CAD build for the part. Positions are in the model's coordinates, mm. Face numbers are marked on the shaded views. A direction names the side the tool comes from. Round coordinates to 2 decimals unless told otherwise and drop trailing zeros. Write each loop counter-clockwise with the first axis right and the second up, starting at its lowest first coordinate (ties: lowest second). Pieces come first, ordered by that corner, then holes. Notation, with made-up numbers: (-30, 66) -> (-24, 66) arc R31 ccw to (-24, 92) -> close; hole circle Ø1 at (26.5, 14.5). An arc over 180 degrees is marked (long way). Put each result on its own line as item: value. Start each with the question number.
1. Saw through at B-B on z = 0. List the corners of the cut face in (x, y), and give its area (3 significant figures).
2. Pull direction Z, two halves, no side cores. Call the marked faces 1, 2 and 3: pulls with the +Z half, pulls with the -Z half, needs draft (parallel to the pull), parting line crosses it, or undercut.
3. Drill centre lines: line 1 (X direction, y = 1.2, z = 0); line 2 (X direction, y = 0.6, z = 1.25); line 3 (Z direction, x = 12, y = 1.6). Where is each one in solid material? Low to high. Write a range as from..to.
4. Flat gauge pins, fed straight in: P1, Ø0.9, axis at y = 2, z = 5.5, coming from the +X side; P2, Ø6, axis at x = 9, z = 1, coming from the +Y side; P3, Ø1, axis at x = 22.5, y = 1, coming from the +Z side. Where does each tip first touch, or does it go through?
5. Saw through at C-C on y = 0.55. List the corners of the cut face in (x, z), and give its area (3 significant figures).
6. 3-axis set-ups, long thin cutter, end or side, ignore diameter. For the marked faces 4, 5 and 6: which of +Z, -Z, +X, -X, +Y, -Y reach the whole face in a straight line?
7. Saw through at A-A on x = 23.5. List the corners of the cut face in (y, z).
8. Saw through at D-D on x = 19. List the corners of the cut face in (y, z).
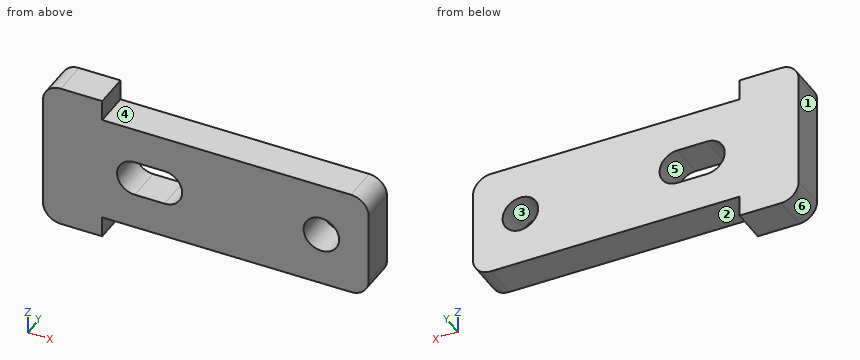
from build123d import *

# Parameters (mm, degrees)
SKETCH_1_R      = 1.5
EXTRUDE_1_DEPTH = 3


with BuildPart() as part:
    # 草图1 → 凸台-拉伸1 (new body)
    with BuildSketch(Plane(origin=(0, 0, 0), x_dir=(1, 0, 0), z_dir=(0, 1, 0))):
        with BuildLine():
            Line((0, 4.75), (0, -4.75))
            ThreePointArc((0, -4.75), (0.439339828, -5.810660172), (1.5, -6.25))
            Line((1.5, -6.25), (5, -6.25))
            Line((5, -6.25), (5, -4.5))
            Line((5, -4.5), (26, -4.5))
            ThreePointArc((26, -4.5), (27.060660172, -4.060660172), (27.5, -3))
            Line((27.5, -3), (27.5, 3))
            ThreePointArc((27.5, 3), (27.060660172, 4.060660172), (26, 4.5))
            Line((26, 4.5), (5, 4.5))
            Line((5, 4.5), (5, 6.25))
            Line((5, 6.25), (1.5, 6.25))
            ThreePointArc((1.5, 6.25), (0.439339828, 5.810660172), (0, 4.75))
        make_face()
        with Locations(Location((23.5, 0, 0), (0, 0, 270))):
            Circle(SKETCH_1_R, mode=Mode.SUBTRACT)
        with BuildLine():
            Line((7.75, 1.5), (10.25, 1.5))
            ThreePointArc((10.25, 1.5), (11.75, 0), (10.25, -1.5))
            Line((10.25, -1.5), (7.75, -1.5))
            ThreePointArc((7.75, -1.5), (6.25, 0), (7.75, 1.5))
        make_face(mode=Mode.SUBTRACT)
    extrude(amount=EXTRUDE_1_DEPTH)


solid = part.part
Return value:
1. outline: (0, 0) -> (6.25, 0) -> (6.25, 3) -> (0, 3) -> close; (11.75, 0) -> (22, 0) -> (22, 3) -> (11.75, 3) -> close; (25, 0) -> (27.5, 0) -> (27.5, 3) -> (25, 3) -> close
1. area: 57.0 mm^2
2. face 1: needs draft
2. face 2: pulls with the -Z half
2. face 3: undercut
3. line 1: x = 0..6.25, 11.75..22, 25..27.5
3. line 2: x = 0..6.92, 11.08..22.67, 24.33..27.5
3. line 3: z = -4.5..4.5
4. P1: stops at x = 5
4. P2: stops at y = 3
4. P3: stops at z = 4.5
5. outline: (0, -4.75) arc R1.5 ccw to (1.5, -6.25) -> (5, -6.25) -> (5, -4.5) -> (26, -4.5) arc R1.5 ccw to (27.5, -3) -> (27.5, 3) arc R1.5 ccw to (26, 4.5) -> (5, 4.5) -> (5, 6.25) -> (1.5, 6.25) arc R1.5 ccw to (0, 4.75) -> close; hole (7.75, -1.5) -> (10.25, -1.5) arc R1.5 ccw to (10.25, 1.5) -> (7.75, 1.5) arc R1.5 ccw to start; hole circle Ø3 at (23.5, 0)
5. area: 241 mm^2
6. face 4: +Z, +X, +Y, -Y
6. face 5: +Y, -Y
6. face 6: -Z, -X, +Y, -Y
7. outline: (0, -4.5) -> (3, -4.5) -> (3, -1.5) -> (0, -1.5) -> close; (0, 1.5) -> (3, 1.5) -> (3, 4.5) -> (0, 4.5) -> close
8. outline: (0, -4.5) -> (3, -4.5) -> (3, 4.5) -> (0, 4.5) -> close
